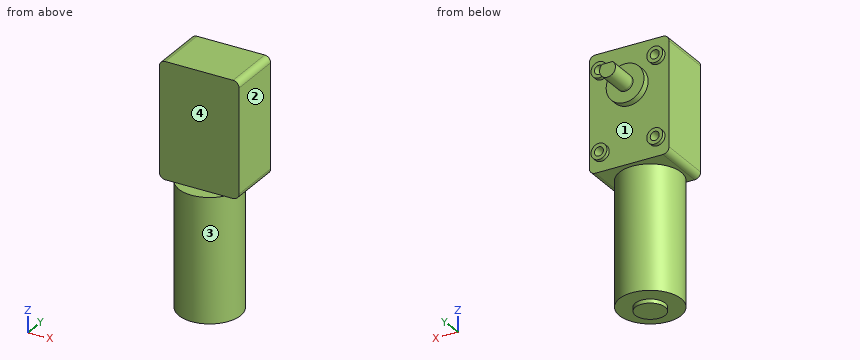
from build123d import *

# Parameters (mm, degrees)
BOSS_EXTRUDE2_DEPTH      = 27
SKETCH2_R                = 4
BOSS_EXTRUDE3_DEPTH      = 2
SKETCH3_R                = 9.5
BOSS_EXTRUDE4_DEPTH      = 3.5
SKETCH4_R                = 4
BOSS_EXTRUDE5_DEPTH      = 1
BOSS_EXTRUDE6_DEPTH      = 14
M4_CLEARANCE_HOLE1_D     = 4.5
M4_CLEARANCE_HOLE1_DEPTH = 9
M4_CLEARANCE_HOLE1_TIP   = 1.351936393
SKETCH8_R                = 15.5
BOSS_EXTRUDE7_DEPTH      = 62
SKETCH9_R                = 7.5
BOSS_EXTRUDE8_DEPTH      = 2


with BuildPart() as part:
    # Sketch1 → Boss-Extrude2 (new body)
    with BuildSketch(Plane(origin=(0, 0, 0), x_dir=(0, 0, -1), z_dir=(0, 1, 0))):
        with BuildLine():
            Line((3, 0), (55, 0))
            ThreePointArc((55, 0), (57.121320344, 0.878679656), (58, 3))
            Line((58, 3), (58, 37))
            ThreePointArc((58, 37), (57.121320344, 39.121320344), (55, 40))
            Line((55, 40), (3, 40))
            ThreePointArc((3, 40), (0.878679656, 39.121320344), (0, 37))
            Line((0, 37), (0, 3))
            ThreePointArc((0, 3), (0.878679656, 0.878679656), (3, 0))
        make_face()
    extrude(amount=BOSS_EXTRUDE2_DEPTH)

    # Sketch2 → Boss-Extrude3 (add)
    with BuildSketch(Plane(origin=(0, 27, 0), x_dir=(1, 0, 0), z_dir=(0, 1, 0))):
        with Locations((-34, 9)):
            Circle(SKETCH2_R)
        with Locations((-6, 9)):
            Circle(SKETCH2_R)
        with Locations((-6, 49)):
            Circle(SKETCH2_R)
        with Locations((-34, 49)):
            Circle(SKETCH2_R)
    extrude(amount=BOSS_EXTRUDE3_DEPTH)

    # Sketch3 → Boss-Extrude4 (add)
    with BuildSketch(Plane(origin=(0, 27, 0), x_dir=(1, 0, 0), z_dir=(0, 1, 0))):
        with Locations((-20, 20)):
            Circle(SKETCH3_R)
    extrude(amount=BOSS_EXTRUDE4_DEPTH)

    # Sketch4 → Boss-Extrude5 (add)
    with BuildSketch(Plane(origin=(0, 30.5, 0), x_dir=(1, 0, 0), z_dir=(0, 1, 0))):
        with Locations((-20, 20)):
            Circle(SKETCH4_R)
    extrude(amount=BOSS_EXTRUDE5_DEPTH)

    # Sketch5 → Boss-Extrude6 (add)
    with BuildSketch(Plane(origin=(0, 31.5, 0), x_dir=(1, 0, 0), z_dir=(0, 1, 0))):
        with BuildLine():
            Line((-22.645751311, 17), (-17.354248689, 17))
            ThreePointArc((-17.354248689, 17), (-20, 24), (-22.645751311, 17))
        make_face()
    extrude(amount=BOSS_EXTRUDE6_DEPTH)

    # M4 Clearance Hole1
    with Locations(Plane(origin=(0, 29, 0), x_dir=(1, 0, 0), z_dir=(0, 1, 0))):
        with Locations((-34, 9), (-34, 49), (-6, 49), (-6, 9)):
            Hole(M4_CLEARANCE_HOLE1_D / 2, depth=M4_CLEARANCE_HOLE1_DEPTH)
            with Locations((0, 0, -(M4_CLEARANCE_HOLE1_DEPTH + M4_CLEARANCE_HOLE1_TIP / 2))):  # 118° drill point
                Cone(0, M4_CLEARANCE_HOLE1_D / 2, M4_CLEARANCE_HOLE1_TIP, mode=Mode.SUBTRACT)

    # Sketch8 → Boss-Extrude7 (add)
    with BuildSketch(Plane(origin=(0, 0, -58), x_dir=(-1, 0, 0), z_dir=(0, 0, -1))):
        with Locations((20, 9)):
            Circle(SKETCH8_R)
    extrude(amount=BOSS_EXTRUDE7_DEPTH)

    # Sketch9 → Boss-Extrude8 (add)
    with BuildSketch(Plane(origin=(0, 0, -120), x_dir=(-1, 0, 0), z_dir=(0, 0, -1))):
        with Locations((20, 9)):
            Circle(SKETCH9_R)
    extrude(amount=BOSS_EXTRUDE8_DEPTH)


solid = part.part
The model under review builds one solid part; all positions refer to its coordinate system, in mm. Face numbers are marked on the shaded views. A direction names the side the tool comes from. Give positions to 0.01 mm unless a question says otherwise; leave off trailing zeros. Write each loop counter-clockwise with the first axis right and the second up, starting at its lowest first coordinate (ties: lowest second). Pieces come first, ordered by that corner, then holes.
1. Add section D-D, the plane y = 4.5. Write out the cut boundary in (x, z), plus the area to 3 significant figures.
2. Tool access review of the marked faces 1, 2, 3 and 4: name each direction out of +Z, -Z, +X, -X, +Y, -Y from which nothing blocks a thin tool from reaching the whole face with its end or side.
3. Add section C-C, the plane z = -73. Write out the cut boundary in (x, y).
4. Add section B-B, the plane y = 42.5. Write out the cut boundary in (x, z), plus the area to 3 significant figures.
5. Add section A-A, the plane x = -20. Write out the cut boundary in (y, z), plus the area to 3 significant figures.
6. Wall thickness on L1, parallel to Z at x = -34, y = 25.25; L2, parallel to X at y = 25.5, z = -49; L3, parallel to X at y = 27.5, z = -49: over which ranges is each line inside the solid? List them lowest first.
7. For P1, Ø10, axis at x = -6.5, y = 6.5, coming from the -Z side; P2, Ø5, axis at x = -6, z = -49, coming from the +Y side; P3, Ø1, axis at y = 15.5, z = -77, coming from the -X side, all flat-tipped, find the tip position at first contact; note any pin that passes through.
Worked answers:
1. outline: (-40, -55) arc R3 ccw to (-37, -58) - (-34.83, -58) - (-34.83, -120) - (-26, -120) - (-26, -122) - (-14, -122) - (-14, -120) - (-5.17, -120) - (-5.17, -58) - (-3, -58) arc R3 ccw to (0, -55) - (0, -3) arc R3 ccw to (-3, 0) - (-37, 0) arc R3 ccw to (-40, -3) - close
1. area: 4,180 mm2
2. face 1: +Y
2. face 2: +Z, -Z, +X, +Y, -Y
2. face 3: -Z
2. face 4: +Z, +X, -X, -Y
3. outline: circle Ø31 at (-20, 9)
4. outline: (-22.65, -17) arc R4 ccw (long way) to (-17.35, -17) - close
4. area: 46.6 mm2
5. outline: (-6.5, -120) - (1.5, -120) - (1.5, -122) - (16.5, -122) - (16.5, -120) - (24.5, -120) - (24.5, -58) - (27, -58) - (27, -29.5) - (30.5, -29.5) - (30.5, -24) - (45.5, -24) - (45.5, -17) - (31.5, -17) - (31.5, -16) - (30.5, -16) - (30.5, -10.5) - (27, -10.5) - (27, 0) - (0, 0) - (0, -58) - (-6.5, -58) - close
5. area: 3,690 mm2
6. L1: z = -58 to -51.25, -46.75 to -11.25, -6.75 to 0
6. L2: x = -40 to -36.25, -31.75 to -8.25, -3.75 to 0
6. L3: x = -38 to -36.25, -31.75 to -30, -10 to -8.25, -3.75 to -2
7. P1: stops at z = -120
7. P2: stops at y = 29
7. P3: stops at x = -34.29
